```python
from build123d import *

# Parameters (mm, degrees)
F1_DEPTH = 10


with BuildPart() as f1:
    # F0 (on Top) → F1 (new body)
    with BuildSketch(Plane.XY):
        Polygon((22.5, 7.5), (22.5, 15), (0, 15), (0, 0), (7.5, 0), (7.5, 7.5), align=None)
    extrude(amount=F1_DEPTH)

    # F2 (on face) → F3 (revolve, cut)
    with BuildSketch(Plane.XZ.offset(-7.5)):
        with BuildLine():
            Line((15, 2.5), (15, 7.5))
            ThreePointArc((15, 7.5), (12.5, 5), (15, 2.5))
        make_face()
    revolve(axis=Axis((15, 7.5, 5), (0, 0, -1)), mode=Mode.SUBTRACT)

    # F4: F1 across plane


with BuildPart() as f1_1:
    add(f1.part)
    add(f1.part.mirror(Plane.XZ))


solid = f1_1.part
```
Check sheet for the modelled part. Datum: model origin and axes. Units: mm. A direction names the side the tool comes from. Coordinates: 2 decimals unless noted, no trailing zeros. Write each loop counter-clockwise with the first axis right and the second up, starting at its lowest first coordinate (ties: lowest second). Pieces come first, ordered by that corner, then holes. Notation, with made-up numbers: (35, 73) - (81, 73) arc R29 cw to (81, 111) - close; hole circle Ø6 at (33, 79.25). An arc over 180 degrees is marked (long way). One line per question, with ' | ' between items.
Item 1: Thickness scan on line 1 (Y direction, x = 7.75, z = 8); line 2 (X direction, y = -0.75, z = 9.75); line 3 (X direction, y = 8.25, z = 5.25). Record the ranges inside material, lowest first. Write a range as [from, to].
Determined:
line 1: y = [-15, -7.5], [7.5, 15] | line 2: x = [0, 7.5] | line 3: x = [0, 12.63], [17.37, 22.5]
Item 2: Access from +Z, -Z, +X, -X, +Y, -Y to the whole of each face (thin tool, end or side, straight path). Record for faces 4 (the face through (22.5, -11, 5)), 5 (the face through (17, -7.5, 3)).
Determined:
face 4: +Z, -Z, +X, +Y, -Y | face 5: +Z, -Z, +X
Item 3: Sectioned sample at D-D on y = 8.25. Record the boundary of the cut face in (x, z), plus the area to 3 significant figures.
Determined:
outline: (0, 0) - (22.5, 0) - (22.5, 10) - (0, 10) - close; hole circle Ø4.77 at (15, 5) | area: 207 mm2
Item 4: Gauge pin test, flat ends, axial feed: P1, Ø8, axis at x = 5, y = -4.5, coming from the -Z side; P2, Ø6, axis at y = 2, z = 4, coming from the +X side. Record the tip position at first contact, or that the pin passes through.
Determined:
P1: stops at z = 0 | P2: stops at x = 7.5
Item 5: Sectioned sample at C-C on x = 13. Record the boundary of the cut face in (y, z), plus the area to 3 significant figures.
Determined:
outline: (-15, 0) - (-7.5, 0) - (-7.5, 3.5) arc R1.5 cw to (-7.5, 6.5) - (-7.5, 10) - (-15, 10) - close; (7.5, 0) - (15, 0) - (15, 10) - (7.5, 10) - (7.5, 6.5) arc R1.5 cw to (7.5, 3.5) - close | area: 143 mm2
Item 6: Mould release check, pull along Y, two halves, no side actions. Record for faces 1 (the face through (11, -15, 5)), 2 (the face through (7.5, 0, 5)), 3 (the face through (22.5, 11, 5)): pulls with the +Y half, pulls with the -Y half, needs draft (parallel to the pull), parting line crosses it, or undercut.
Determined:
face 1: pulls with the -Y half | face 2: undercut | face 3: needs draft
Item 7: Sectioned sample at A-A on x = 19. Record the boundary of the cut face in (y, z), plus the area to 3 significant figures.
Determined:
outline: (-15, 0) - (-7.5, 0) - (-7.5, 10) - (-15, 10) - close; (7.5, 0) - (15, 0) - (15, 10) - (7.5, 10) - close | area: 150 mm2
Item 8: Sectioned sample at B-B on z = 5. Record the boundary of the cut face in (x, y), plus the area to 3 significant figures.
Determined:
outline: (0, -15) - (22.5, -15) - (22.5, -7.5) - (17.5, -7.5) arc R2.5 cw to (12.5, -7.5) - (7.5, -7.5) - (7.5, 7.5) - (12.5, 7.5) arc R2.5 cw to (17.5, 7.5) - (22.5, 7.5) - (22.5, 15) - (0, 15) - close | area: 430 mm2
